```python
from build123d import *

# Parameters (mm, degrees)
SKETCH1_W           = 115
SKETCH1_H           = 85
BOSS_EXTRUDE1_DEPTH = 60
SKETCH2_W           = 100
SKETCH2_H           = 70
CUT_EXTRUDE1_DEPTH  = 57.5
SKETCH3_W           = 75
SKETCH3_H           = 3.5
CUT_EXTRUDE2_DEPTH  = 109
SKETCH4_W           = 74.99639209
SKETCH4_H           = 45
CUT_EXTRUDE3_DEPTH  = 7.5


with BuildPart() as part:
    # Sketch1 → Boss-Extrude1 (new body)
    with BuildSketch(Plane(origin=(0, 0, 0), x_dir=(1, 0, 0), z_dir=(0, 1, 0))):
        with Locations((57.5, 42.5)):
            Rectangle(SKETCH1_W, SKETCH1_H)
    extrude(amount=BOSS_EXTRUDE1_DEPTH)

    # Sketch2 → Cut-Extrude1 (cut)
    with BuildSketch(Plane(origin=(0, 60, 0), x_dir=(1, 0, 0), z_dir=(0, 1, 0))):
        with Locations((57.5, 42.5)):
            Rectangle(SKETCH2_W, SKETCH2_H)
    extrude(amount=-CUT_EXTRUDE1_DEPTH, mode=Mode.SUBTRACT)

    # Sketch3 → Cut-Extrude2 (cut)
    with BuildSketch(Plane.ZY):
        with Locations((-42.5, 55.75)):
            Rectangle(SKETCH3_W, SKETCH3_H)
    extrude(amount=-CUT_EXTRUDE2_DEPTH, mode=Mode.SUBTRACT)

    # Sketch4 → Cut-Extrude3 (cut)
    with BuildSketch(Plane.ZY):
        with Locations((-42.501803955, 31.5)):
            Rectangle(SKETCH4_W, SKETCH4_H)
    extrude(amount=-CUT_EXTRUDE3_DEPTH, mode=Mode.SUBTRACT)


solid = part.part
```
Source: CAD feature listing. Evaluate the final solid. Frame: model axes, mm. A direction names the side the tool comes from. Give positions to 0.01 mm unless a question says otherwise; leave off trailing zeros. Write each loop counter-clockwise with the first axis right and the second up, starting at its lowest first coordinate (ties: lowest second). Pieces come first, ordered by that corner, then holes. Notation, with made-up numbers: (14.25, 1) - (45.25, 1) arc R18 cw to (45.25, 33) - close; hole circle Ø9 at (77.25, 6.5). An arc over 180 degrees is marked (long way). One line per item, written item: value. Start each with the question number.
Q1. Material intervals for probe 1 along Z at (x, y) = (76, 56.5); probe 2 along Y at (x, z) = (11, -5.5); probe 3 along X at (y, z) = (6, -26.5), sorted ascending. Write a range as from..to.
Q2. Section query C-C, the plane y = 38.5. Return the cut outline in (x, z), then the cut area to 3 significant figures.
Q3. First-contact query: pin 1 Ø1 at (y, z) = (47, -15) entering from -X; pin 2 Ø0.7 at (y, z) = (42.5, -6.5) entering from -X; pin 3 Ø8 at (x, z) = (93.5, -12) entering from +Y. Flat tips, straight axial feed; report the tip coordinate or a pass-through.
Q4. Section query A-A, the plane z = -47.5. Return the cut outline in (x, y).
Q5. Draft query along Y for faces 4 (the face through (57, 60, -5)), 5 (the face through (57, 59, -77.5)), 6 (the face through (58, 54, -7)). Return one class per face: +Y half, -Y half, draft (parallel to the pull), parting line (faces both ways), or undercut.
Q6. Section query B-B, the plane x = 82. Return the cut outline in (y, z), then the cut area to 3 significant figures.
Q7. Set-up query: faces 1 (the face through (57, 30, -85)), 2 (the face through (57, 2.5, -43)), 3 (the face through (4, 9, -43)). Return all of +Z, -Z, +X, -X, +Y, -Y with unobstructed straight access to the full face (end or side cutting, diameter ignored); none if empty.
Answer:
1. probe 1: z = -85..-80, -5..0
1. probe 2: y = 0..54, 57.5..60
1. probe 3: x = 0..7.5, 107.5..115
2. outline: (0, -85) - (115, -85) - (115, 0) - (0, 0) - (0, -5) - (7.5, -5) - (7.5, -7.5) - (107.5, -7.5) - (107.5, -77.5) - (7.5, -77.5) - (7.5, -80) - (0, -80) - close
2. area: 2,210 mm2
3. pin 1: stops at x = 107.5
3. pin 2: stops at x = 7.5
3. pin 3: stops at y = 2.5
4. outline: (0, 0) - (115, 0) - (115, 60) - (107.5, 60) - (107.5, 57.5) - (109, 57.5) - (109, 54) - (107.5, 54) - (107.5, 2.5) - (7.5, 2.5) - (7.5, 9) - (0, 9) - close; (0, 57.5) - (7.5, 57.5) - (7.5, 60) - (0, 60) - close
5. face 4: +Y half
5. face 5: draft
5. face 6: undercut
6. outline: (0, -85) - (60, -85) - (60, -77.5) - (57.5, -77.5) - (57.5, -80) - (54, -80) - (54, -77.5) - (2.5, -77.5) - (2.5, -7.5) - (54, -7.5) - (54, -5) - (57.5, -5) - (57.5, -7.5) - (60, -7.5) - (60, 0) - (0, 0) - close
6. area: 1,060 mm2
7. face 1: -Z, +X, -X, +Y, -Y
7. face 2: +Y
7. face 3: -X
